Geometry check sheet. Reference: drawing and pictorial views, mm from the part's lowest x, y, z. Give positions to 0.01 mm unless a question says otherwise; leave off trailing zeros. Order: outer loops, then holes, each group sorted by start corner. A loop starts at its lowest first (then second) coordinate and runs counter-clockwise, first axis right, second up. Notation, with made-up numbers: (14.25, 50) -> (60.25, 50) arc R5 cw to (60.25, 54) -> close; hole circle Ø3 at (5, 71). An arc over 180 degrees is marked (long way). Write each question's results on one line, items separated by ' | '. Start each with the question number.
1. Cross-section at B-B, the plane y = 1.95. Enter the section's corners in (x, z).
2. Cross-section at D-D, the plane x = 48.75. Enter the section's corners in (y, z).
3. Depth check by flat-ended pin: pin 1 Ø2.5 at (x, y) = (14.5, 2) entering from +Z; pin 2 Ø10 at (x, z) = (54.5, 30.5) entering from -Y; pin 3 Ø1.5 at (y, z) = (2, 14) entering from +X; pin 4 Ø1.5 at (y, z) = (2.5, 54) entering from +X. Enter the tip coordinate at first touch or a pass-through.
4. Cross-section at C-C, the plane x = 35. Enter the section's corners in (y, z), then the cut area to 3 significant figures.
5. Cross-section at A-A, the plane z = 35. Enter the section's corners in (x, y).
6. Material ranges on L1, parallel to X at y = 2.6, z = 35; L2, parallel to Z at x = 54, y = 1.2; L3, parallel to Z at x = 53.5, y = 3, recorded low to high. Write a range as from..to.
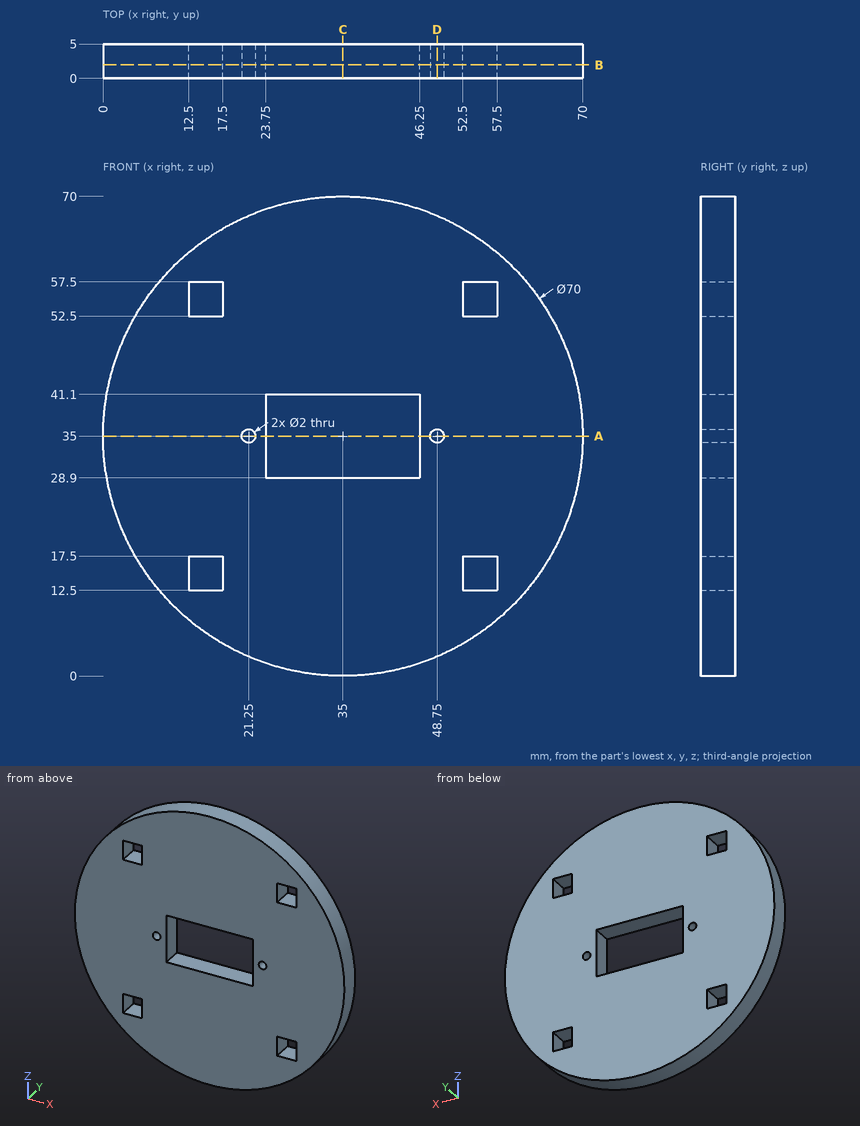
Results below:
1) outline: circle Ø70 at (35, 35); hole (12.5, 12.5) -> (17.5, 12.5) -> (17.5, 17.5) -> (12.5, 17.5) -> close; hole (12.5, 52.5) -> (17.5, 52.5) -> (17.5, 57.5) -> (12.5, 57.5) -> close; hole circle Ø2 at (21.25, 35); hole (23.75, 28.9) -> (46.25, 28.9) -> (46.25, 41.1) -> (23.75, 41.1) -> close; hole circle Ø2 at (48.75, 35); hole (52.5, 12.5) -> (57.5, 12.5) -> (57.5, 17.5) -> (52.5, 17.5) -> close; hole (52.5, 52.5) -> (57.5, 52.5) -> (57.5, 57.5) -> (52.5, 57.5) -> close
2) outline: (0, 2.81) -> (5, 2.81) -> (5, 34) -> (0, 34) -> close; (0, 36) -> (5, 36) -> (5, 67.19) -> (0, 67.19) -> close
3) pin 1: stops at z = 64.23 | pin 2: stops at y = 0 | pin 3: stops at x = 63.55 | pin 4: stops at x = 64.87
4) outline: (0, 0) -> (5, 0) -> (5, 28.9) -> (0, 28.9) -> close; (0, 41.1) -> (5, 41.1) -> (5, 70) -> (0, 70) -> close | area: 289 mm²
5) outline: (0, 0) -> (20.25, 0) -> (20.25, 5) -> (0, 5) -> close; (22.25, 0) -> (23.75, 0) -> (23.75, 5) -> (22.25, 5) -> close; (46.25, 0) -> (47.75, 0) -> (47.75, 5) -> (46.25, 5) -> close; (49.75, 0) -> (70, 0) -> (70, 5) -> (49.75, 5) -> close
6) L1: x = 0..20.25, 22.25..23.75, 46.25..47.75, 49.75..70 | L2: z = 5.61..12.5, 17.5..52.5, 57.5..64.39 | L3: z = 5.29..12.5, 17.5..52.5, 57.5..64.71
